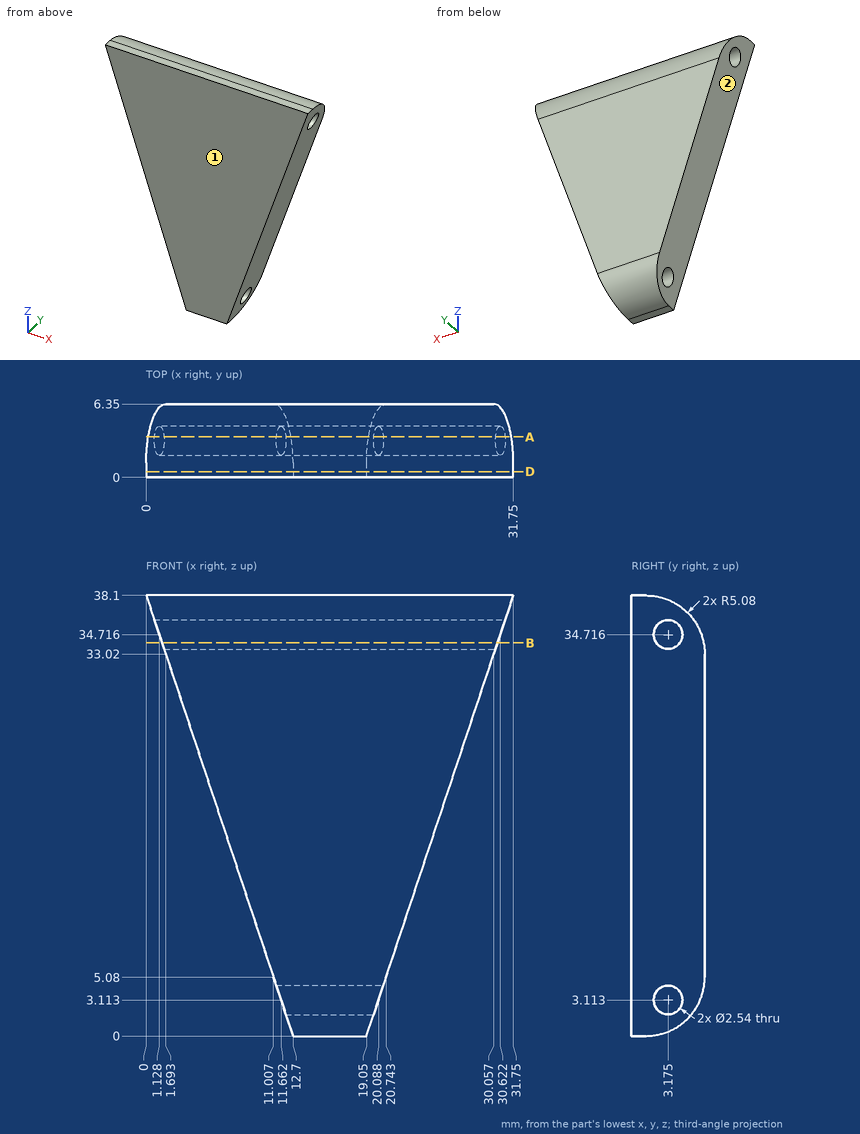
Source: three-view drawing plus pictorial views. Frame: mm from the lowest corner of the part. Round coordinates to 2 decimals unless told otherwise and drop trailing zeros. Loops run counter-clockwise (first coordinate to the right, second up) from the corner with the lowest first, then second, coordinate; pieces in that order, holes last.
1. Mould query, pull axis X, two halves, no side actions, for the marked faces 1 and 2. Classes: released by +X, released by -X, zero draft, split by the parting line, or undercut.
2. Section query D-D on y = 0.5. Output: boundary loops of the cut face in (x, z).
3. Contact query for flat-ended pins moving along their axis: pin 1 (1.5 mm diameter, centred on x = 25.5, y = 5.5, fed in from +Z); pin 2 (3 mm diameter, centred on y = 1.5, z = 26.5, fed in from +X); pin 3 (1.5 mm diameter, centred on x = 13, y = 2, fed in from -Z); pin 4 (1 mm diameter, centred on y = 3, z = 12, fed in from +X). Output: stop coordinate, or through.
4. Section query A-A on y = 3.5. Output: boundary loops of the cut face in (x, z) (1 decimal), and give its area (3 significant figures).
5. Ray query, L1, parallel to Z at x = 15, y = 3 (1 decimal); L2, parallel to Z at x = 15, y = 2.75; L3, parallel to X at y = 1.75, z = 36. Return the intervals inside material, ascending.
6. Section query B-B on z = 34. Output: boundary loops of the cut face in (x, y) (1 decimal).
Answers below:
1. face 1: zero draft
1. face 2: released by -X
2. outline: (0, 38.1) - (12.7, 0) - (19.05, 0) - (31.75, 38.1) - close
3. pin 1: stops at z = 36.72
3. pin 2: stops at x = 28.38
3. pin 3: stops at z = 0
3. pin 4: stops at x = 23.22
4. outline: (0.2, 37.6) - (0.7, 35.9) - (31, 35.9) - (31.6, 37.6) - close; (1.5, 33.5) - (11.3, 4.3) - (20.5, 4.3) - (30.2, 33.5) - close; (12.1, 1.9) - (12.5, 0.5) - (19.2, 0.5) - (19.7, 1.9) - close
4. area: 613 mm2
5. L1: z = 0.3 to 1.9, 4.4 to 33.5, 36 to 37.8
5. L2: z = 0.22 to 1.92, 4.31 to 33.52, 35.91 to 37.88
5. L3: x = 0.7 to 31.05
6. outline: (1.4, 0) - (30.4, 0) - (30.4, 2.1) - (1.4, 2.1) - close; (1.4, 4.2) - (30.4, 4.2) - (30.4, 6.3) - (1.4, 6.3) - close
